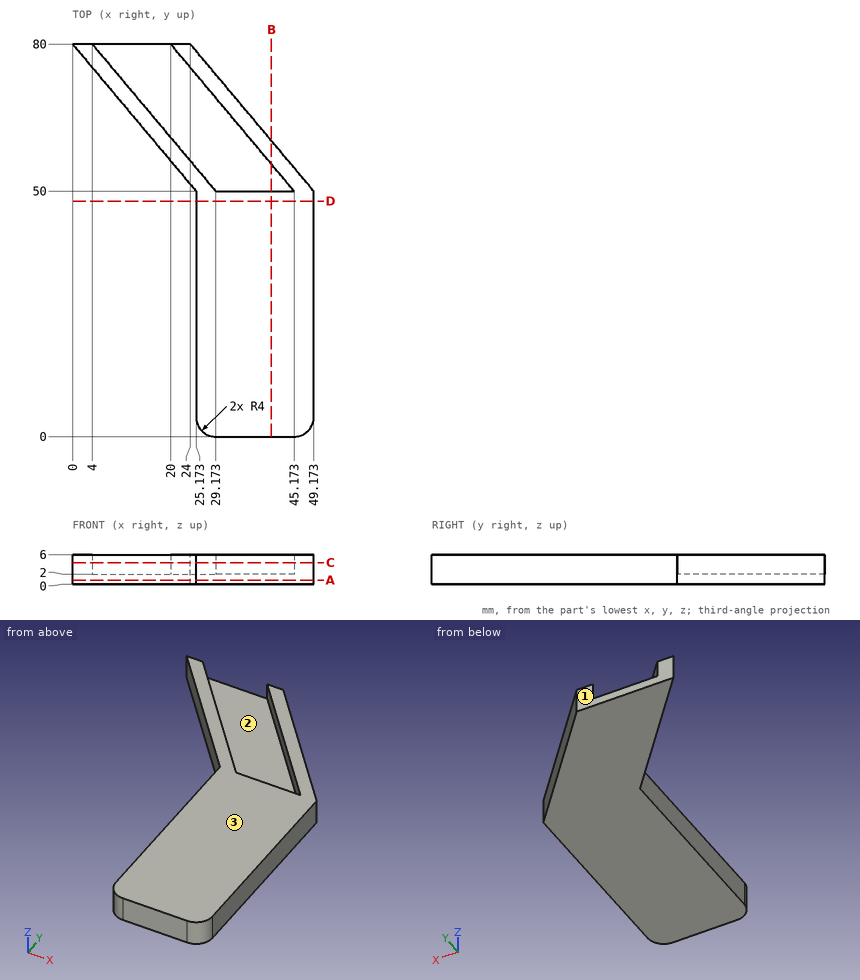
Study the drawing (mm; zero at the part's minimum x, y, z) and answer. Give positions to 0.01 mm unless a question says otherwise; leave off trailing zeros. Write each loop counter-clockwise with the first axis right and the second up, starting at its lowest first coordinate (ties: lowest second). Pieces come first, ordered by that corner, then holes. Notation, with made-up numbers: (41.5, 27) - (67.5, 27) arc R22 cw to (67.5, 53) - close; hole circle Ø10 at (72.25, -25.5). An arc over 180 degrees is marked (long way). One line per question, with ' | ' between items. Start each with the question number.
1. Straight lines are drawn through the part: line 1 (X direction, y = 19, z = 0.5); line 2 (X direction, y = 73, z = 4.6); line 3 (X direction, y = 56, z = 4.3). For each, find the intervals that lie inside material, in ascending order.
2. Section D-D, the plane y = 48 is taken. Determine the outline of the cut face in (x, z).
3. Determine the mould class of the marked faces 1, 2 and 3 for opening direction Y: +Y half, -Y half, draft (parallel to the pull), parting line (faces both ways), or undercut.
4. Section C-C, the plane z = 4.4 is taken. Determine the outline of the cut face in (x, y), then the cut area to 3 significant figures.
5. Section B-B, the plane x = 40.5 is taken. Determine the outline of the cut face in (y, z).
6. Given P1, Ø3, axis at y = 57.5, z = 1, coming from the +X side; P2, Ø1, axis at x = 15.5, z = 3, coming from the -Y side; P3, Ø1.2, axis at x = 40.5, z = 3.5, coming from the +Y side, each flat-ended and moving along its own axis, determine where each tip first touches the part or whether it passes through.
7. Section A-A, the plane z = 0.8 is taken. Determine the outline of the cut face in (x, y), then the cut area to 3 significant figures.
Result:
1) line 1: x = 25.17 to 49.17 | line 2: x = 5.87 to 9.87, 25.87 to 29.87 | line 3: x = 20.14 to 24.14, 40.14 to 44.14
2) outline: (25.17, 0) - (49.17, 0) - (49.17, 6) - (25.17, 6) - close
3) face 1: +Y half | face 2: undercut | face 3: draft
4) outline: (0, 80) - (25.17, 50) - (25.17, 4) arc R4 ccw to (29.17, 0) - (45.17, 0) arc R4 ccw to (49.17, 4) - (49.17, 50) - (24, 80) - (20, 80) - (45.17, 50) - (29.17, 50) - (4, 80) - close | area: 1,430 mm2
5) outline: (0, 0) - (60.34, 0) - (60.34, 6) - (55.57, 6) - (55.57, 2) - (50, 2) - (50, 6) - (0, 6) - close
6) P1: stops at x = 44.14 | P2: stops at y = 60.93 | P3: stops at y = 61.05
7) outline: (0, 80) - (25.17, 50) - (25.17, 4) arc R4 ccw to (29.17, 0) - (45.17, 0) arc R4 ccw to (49.17, 4) - (49.17, 50) - (24, 80) - close | area: 1,910 mm2
